Design review of the part built by this model. Coordinates are the model's own, in mm. A direction names the side the tool comes from. Round coordinates to 2 decimals unless told otherwise and drop trailing zeros. Order: outer loops, then holes, each group sorted by start corner. A loop starts at its lowest first (then second) coordinate and runs counter-clockwise, first axis right, second up. Notation, with made-up numbers: M 0.5,23 L 26.5,23 A27 cw 26.5,39 Z; hole C 73,11 d11. An arc over 180 degrees is marked long. Use a Markdown table: item, result. Add a question column.
(1) Take a section at A-A (y = 0). Write out the cut boundary in (x, z), then the cut area to 3 significant figures.
(2) The part is to be moulded in two halves that separate along Y. For faces 1 (the face through (-0.2, -3.3, 8)), 2 (the face through (-3.47, -15.62, 3.94)), 3 (the face through (-3, 0, 4)), say which applies: released by +Y, released by -Y, zero draft, split by the parting line, or undercut.
(3) Take a section at B-B (z = 3.5). Count the separate pieces of the cut face and the enclosed holes in it, then the cut area to 3 significant figures.
(4) To check wall thickness, follow probe 1 along Y at (x, z) = (0, 2.75); probe 2 along Y at (x, z) = (-6, 6.25); probe 3 along X at (y, z) = (-1, 1). State the ranges of each line that lie inside material, in increasing order. Write a range as from..to.
(5) For pin 1 (4 mm diameter, centred on y = -4.5, z = 7, fed in from -X); pin 2 (2.5 mm diameter, centred on x = -5, y = -5, fed in from +Z); pin 3 (1.5 mm diameter, centred on y = 10.5, z = 6.5, fed in from +X), all flat-tipped, find the tip position at first contact; note any pin that passes through.
(6) Machinability: for faces 4 (the face through (-6, -6, 3)), 5 (the face through (-0.2, -3.3, 0)), which of the approach directions +Z, -Z, +X, -X, +Y, -Y give a long, thin tool a straight path to every point of the face, cutting with its end or side? Answer none if there is none.
(7) Take a section at D-D (x = -11). Write out the cut boundary in (y, z).
(8) Take a section at C-C (y = 12). Write out the cut boundary in (x, z).
```python
from build123d import *

# Parameters (mm, degrees)
F0_R     = 16
F1_DEPTH = 8
F3_DEPTH = 5
F4_R     = 3
F5_DEPTH = 25


with BuildPart() as f1:
    # F0 (on Top) → F1 (new body)
    with BuildSketch(Plane.XY):
        Circle(F0_R)
    extrude(amount=F1_DEPTH)

    # F2 (on face) → F3 (cut)
    with BuildSketch(Plane.XY.offset(8)):
        with BuildLine():
            ThreePointArc((6, -1.75), (2.994796, -2.994796), (1.75, -6))
            Line((1.75, -6), (6, -6))
            Line((6, -6), (6, -1.75))
        make_face()
        with BuildLine():
            Line((6, -6), (1.75, -6))
            ThreePointArc((1.75, -6), (6, -10.25), (10.25, -6))
            ThreePointArc((10.25, -6), (9.005204, -2.994796), (6, -1.75))
            Line((6, -1.75), (6, -6))
        make_face()
        with BuildLine():
            Line((-6, -6), (-1.75, -6))
            ThreePointArc((-1.75, -6), (-2.994796, -2.994796), (-6, -1.75))
            Line((-6, -1.75), (-6, -6))
        make_face()
        with BuildLine():
            ThreePointArc((-6, -1.75), (-9.005204, -9.005204), (-1.75, -6))
            Line((-1.75, -6), (-6, -6))
            Line((-6, -6), (-6, -1.75))
        make_face()
        with BuildLine():
            ThreePointArc((1.75, 6), (2.994796, 2.994796), (6, 1.75))
            Line((6, 1.75), (6, 6))
            Line((6, 6), (1.75, 6))
        make_face()
        with BuildLine():
            Line((6, 6), (6, 1.75))
            ThreePointArc((6, 1.75), (9.005204, 2.994796), (10.25, 6))
            ThreePointArc((10.25, 6), (6, 10.25), (1.75, 6))
            Line((1.75, 6), (6, 6))
        make_face()
        with BuildLine():
            ThreePointArc((-1.75, 6), (-9.005204, 9.005204), (-6, 1.75))
            Line((-6, 1.75), (-6, 6))
            Line((-6, 6), (-1.75, 6))
        make_face()
        with BuildLine():
            Line((-6, 6), (-6, 1.75))
            ThreePointArc((-6, 1.75), (-2.994796, 2.994796), (-1.75, 6))
            Line((-1.75, 6), (-6, 6))
        make_face()
    extrude(amount=-F3_DEPTH, mode=Mode.SUBTRACT)

    # F4 (on face) → F5 (cut)
    with BuildSketch(Plane.XY.offset(8)):
        Circle(F4_R)
        with Locations((-12, 0)):
            Circle(F4_R)
        with Locations((0, 12)):
            Circle(F4_R)
        with Locations((12, 0)):
            Circle(F4_R)
        with Locations((0, -12)):
            Circle(F4_R)
    extrude(amount=-F5_DEPTH, mode=Mode.SUBTRACT)


solid = f1.part
```
Verdict:
| question | item | result |
|---|---|---|
| 1 | outline | M -16,0 L -15,0 L -15,8 L -16,8 Z; M -9,0 L -3,0 L -3,8 L -9,8 Z; M 3,0 L 9,0 L 9,8 L 3,8 Z; M 15,0 L 16,0 L 16,8 L 15,8 Z |
| 1 | area | 112 mm^2 |
| 2 | face 1 | zero draft |
| 2 | face 2 | split by the parting line |
| 2 | face 3 | undercut |
| 3 | separate pieces | 1 |
| 3 | enclosed holes | 9 |
| 3 | area | 436 mm^2 |
| 4 | probe 1 | y = -16..-15, -9..-3, 3..9, 15..16 |
| 4 | probe 2 | y = -14.83..-10.25, -1.75..1.75, 10.25..14.83 |
| 4 | probe 3 | x = -15.97..-14.83, -9.17..-2.83, 2.83..9.17, 14.83..15.97 |
| 5 | pin 1 | stops at x = -15.8 |
| 5 | pin 2 | stops at z = 3 |
| 5 | pin 3 | stops at x = 12.69 |
| 6 | face 4 | +Z |
| 6 | face 5 | -Z, +X, -X, +Y, -Y |
| 7 | outline | M -11.62,0 L -2.83,0 L -2.83,8 L -11.62,8 Z; M 2.83,0 L 11.62,0 L 11.62,8 L 2.83,8 Z |
| 8 | outline | M -10.58,0 L -3,0 L -3,8 L -10.58,8 Z; M 3,0 L 10.58,0 L 10.58,8 L 3,8 Z |
